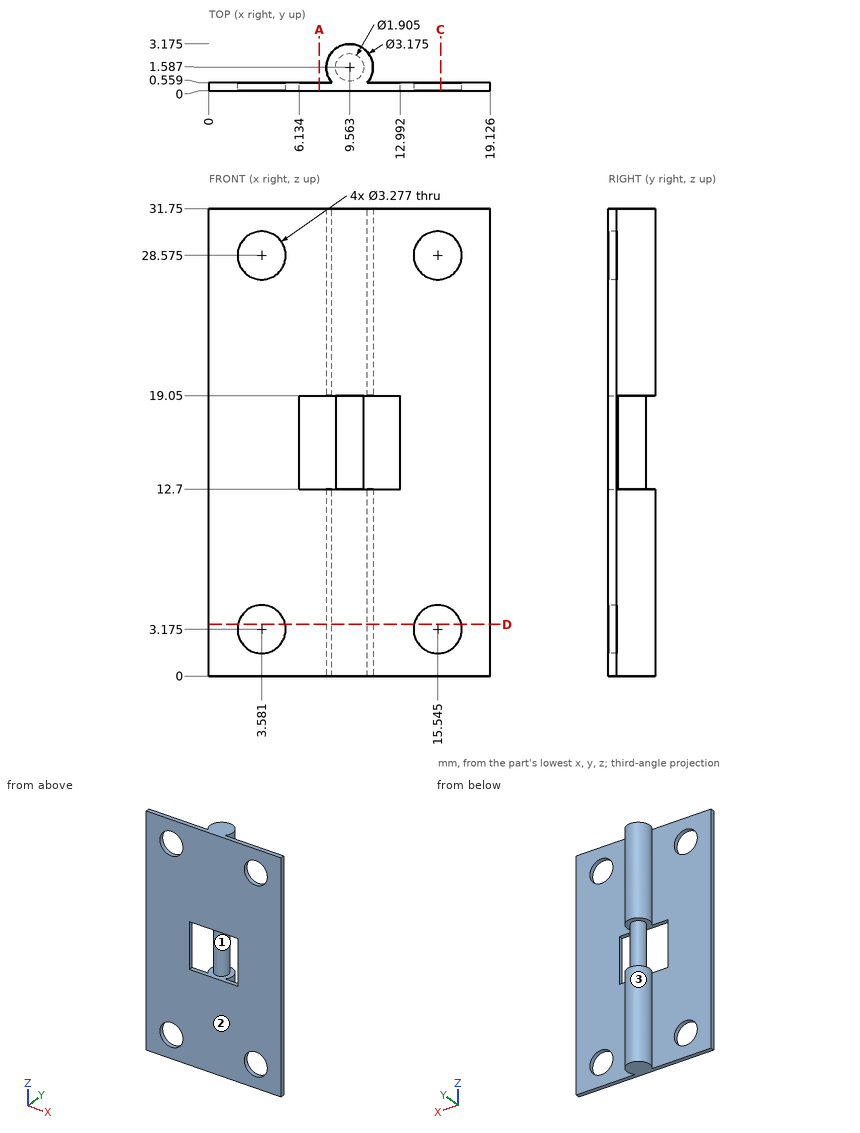
Verification items for this drawing (mm, ordinates from the low corner). Give positions to 0.01 mm unless a question says otherwise; leave off trailing zeros. Loops run counter-clockwise (first coordinate to the right, second up) from the corner with the lowest first, then second, coordinate; pieces in that order, holes last. Notation, with made-up numbers: M 56,72.25 L 79,72.25 A28 cw 79,101.25 Z; hole C 80.5,70.5 d1. An arc over 180 degrees is marked long. Answer as a JSON object with one key per item and string values. Group by question number.
Item 1: Material ranges on L1, parallel to Y at x = 3.25, z = 30.5; L2, parallel to X at y = 1.6, z = 19 (1 decimal); L3, parallel to X at y = 0.9, z = 27.5 (1 decimal), recorded low to high.
Item 2: Sectioned sample at D-D on z = 3.5. Give the number of separate pieces and of enclosed holes in the cut face.
Item 3: Sectioned sample at A-A on x = 7.5. Record the boundary of the cut face in (y, z).
Item 4: Gauge pin test, flat end, axial feed: pin 1 (4 mm diameter, centred on x = 17, z = 21, fed in from +Y). Record the tip position at first contact, or that the pin passes through.
Item 5: Sectioned sample at C-C on x = 15.75. Record the boundary of the cut face in (y, z).
Item 6: Mould release check, pull along Y, two halves, no side actions. Record for the marked faces 1, 2 and 3: pulls with the +Y half, pulls with the -Y half, needs draft (parallel to the pull), parting line crosses it, or undercut.
Findings below:
{
 "1": {"L1": "0 to 0.56", "L2": "8.6 to 10.5", "L3": "8.1 to 11"},
 "2": {"separate pieces": "3", "enclosed holes": "0"},
 "3": {"outline": "M 0,0 L 0.56,0 L 0.56,12.7 L 0,12.7 Z; M 0,19.05 L 0.56,19.05 L 0.56,31.75 L 0,31.75 Z"},
 "4": {"pin 1": "y = 0.56"},
 "5": {"outline": "M 0,0 L 0.56,0 L 0.56,1.55 L 0,1.55 Z; M 0,4.8 L 0.56,4.8 L 0.56,26.95 L 0,26.95 Z; M 0,30.2 L 0.56,30.2 L 0.56,31.75 L 0,31.75 Z"},
 "6": {"face 1": "parting line crosses it", "face 2": "pulls with the -Y half", "face 3": "undercut"}
}
